Verification items for the finished model (mm, model axes). Coordinates: 2 decimals unless noted, no trailing zeros. Order: outer loops, then holes, each group sorted by start corner. A loop starts at its lowest first (then second) coordinate and runs counter-clockwise, first axis right, second up. Notation, with made-up numbers: M 69,22.5 L 77,22.5 A15 ccw 77,38.5 Z; hole C 65.5,5 d11. An arc over 180 degrees is marked long. Use one line per item in the form item = value. Start each with the question number.
```python
from build123d import *

# Parameters (mm, degrees)
SKETCH1_W           = 17.8
SKETCH1_H           = 8
BOSS_EXTRUDE1_DEPTH = 2.35
SKETCH2_R           = 2.26
CUT_EXTRUDE1_DEPTH  = 20.656105922
FILLET1_R           = 4


with BuildPart() as part:
    # Sketch1 → Boss-Extrude1 (new body)
    with BuildSketch(Plane(origin=(0, 0, 0), x_dir=(1, 0, 0), z_dir=(0, 1, 0))):
        with Locations((8.9, 4)):
            Rectangle(SKETCH1_W, SKETCH1_H)
    extrude(amount=BOSS_EXTRUDE1_DEPTH)

    # Sketch2 → Cut-Extrude1 (cut, through all)
    with BuildSketch(Plane(origin=(0, 2.35, 0), x_dir=(1, 0, 0), z_dir=(0, 1, 0))):
        with Locations(Location((4, 4, 0), (0, 0, 270))):
            Circle(SKETCH2_R)
        with Locations(Location((13.8, 4, 0), (0, 0, 270))):
            Circle(SKETCH2_R)
    extrude(amount=-CUT_EXTRUDE1_DEPTH, mode=Mode.SUBTRACT)

    # Fillet1
    fillet1_edges = [part.edges().sort_by_distance(p)[0] for p in [
        (17.8, 1.175, 0),
        (0, 1.175, 0),
        (17.8, 1.175, -8),
        (0, 1.175, -8),
    ]]
    fillet(fillet1_edges, radius=FILLET1_R - 0.0001)  # a hair under: the kernel refuses the full size


solid = part.part
```
1. Material ranges on line 1 along X through (y, z) = (0.65, -4); line 2 along X through (y, z) = (1.2, -4.5); line 3 along Z through (x, y) = (2, 1.85), recorded low to high.
2. Cross-section at C-C on x = 15.25. Enter the section's corners in (y, z), and give its area (3 significant figures).
3. Release check for a two-part mould opening along Z. For faces 1 (the cylindrical face through (5.527, 1.191, -5.666)), 2 (the cylindrical face through (1.141, 1.191, -1.203)), 3 (the cylindrical face through (1.141, 1.191, -6.797)) record: pulls with the +Z half, pulls with the -Z half, needs draft (parallel to the pull), parting line crosses it, or undercut.
4. Cross-section at D-D on z = -2.25. Enter the section's corners in (x, y).
5. Cross-section at A-A on z = -4.5. Enter the section's corners in (x, y), and give its area (3 significant figures).
6. Cross-section at B-B on y = 2. Give the number of separate pieces and of enclosed holes in the cut face, and give its area (3 significant figures).
Final values:
q1.line_1 = 0 to 1.74, 6.26 to 11.54, 16.06 to 17.8
q1.line_2 = 0.03 to 1.8, 6.2 to 11.6, 16 to 17.77
q1.line_3 = -7.46 to -5.05, -2.95 to -0.54
q2.outline = M 0,-7.73 L 2.35,-7.73 L 2.35,-5.73 L 0,-5.73 Z; M 0,-2.27 L 2.35,-2.27 L 2.35,-0.27 L 0,-0.27 Z
q2.area = 9.37 mm2
q3.face_1 = undercut
q3.face_2 = pulls with the +Z half
q3.face_3 = pulls with the -Z half
q4.outline = M 0.4,0 L 2.57,0 L 2.57,2.35 L 0.4,2.35 Z; M 5.43,0 L 12.37,0 L 12.37,2.35 L 5.43,2.35 Z; M 15.23,0 L 17.4,0 L 17.4,2.35 L 15.23,2.35 Z
q5.outline = M 0.03,0 L 1.8,0 L 1.8,2.35 L 0.03,2.35 Z; M 6.2,0 L 11.6,0 L 11.6,2.35 L 6.2,2.35 Z; M 16,0 L 17.77,0 L 17.77,2.35 L 16,2.35 Z
q5.area = 21.0 mm2
q6.separate_pieces = 1
q6.enclosed_holes = 2
q6.area = 96.6 mm2
